from build123d import *

# Parameters (mm, degrees)
F1_DEPTH = 9.525
F3_D     = 2.7178


with BuildPart() as f1:
    # F0 (on Top) → F1 (new body)
    with BuildSketch(Plane.XY):
        with BuildLine():
            Line((161.925, -95.25), (161.925, 95.25))
            ThreePointArc((161.925, 95.25), (160.065128, 99.740128), (155.575, 101.6))
            Line((155.575, 101.6), (34.925, 101.6))
            ThreePointArc((34.925, 101.6), (30.434872, 99.740128), (28.575, 95.25))
            Line((28.575, 95.25), (28.575, 63.5))
            ThreePointArc((28.575, 63.5), (13.696024, 27.578976), (-22.225, 12.7))
            Line((-22.225, 12.7), (-155.575, 12.7))
            ThreePointArc((-155.575, 12.7), (-160.065128, 10.840128), (-161.925, 6.35))
            Line((-161.925, 6.35), (-161.925, -95.25))
            ThreePointArc((-161.925, -95.25), (-160.065128, -99.740128), (-155.575, -101.6))
            Line((-155.575, -101.6), (155.575, -101.6))
            ThreePointArc((155.575, -101.6), (160.065128, -99.740128), (161.925, -95.25))
        make_face()
        with BuildLine():
            Line((47.371, 9.652), (142.875, 9.652))
            ThreePointArc((142.875, 9.652), (145.030261, 8.759261), (145.923, 6.604))
            Line((145.923, 6.604), (145.923, -22.352))
            ThreePointArc((145.923, -22.352), (145.030261, -24.507261), (142.875, -25.4))
            Line((142.875, -25.4), (47.371, -25.4))
            ThreePointArc((47.371, -25.4), (45.215739, -24.507261), (44.323, -22.352))
            Line((44.323, -22.352), (44.323, 6.604))
            ThreePointArc((44.323, 6.604), (45.215739, 8.759261), (47.371, 9.652))
        make_face(mode=Mode.SUBTRACT)
    extrude(amount=-F1_DEPTH)

    # F3 (through all)
    with Locations(Plane.XY):
        with Locations((118.999, -56.134), (118.999, 14.732), (118.999, 68.834), (71.247, 68.834), (71.247, 14.732), (71.247, -56.134), (21.717, -60.706), (21.717, -91.44), (-3.683, -60.706), (-3.683, -91.44), (-29.083, -60.706), (-29.083, -91.44), (-54.483, -91.44), (-54.483, -60.706), (-66.929, -52.832), (-66.929, -21.082), (-92.329, -52.832), (-92.329, -21.082), (-124.079, -52.832), (-124.079, -21.082), (-149.479, -52.832), (-149.479, -21.082)):
            Hole(F3_D / 2)


solid = f1.part
Input: part model. Units: mm. Frame: model coordinates. A direction names the side the tool comes from. Give positions to 0.01 mm unless a question says otherwise; leave off trailing zeros. Loops run counter-clockwise (first coordinate to the right, second up) from the corner with the lowest first, then second, coordinate; pieces in that order, holes last. Notation, with made-up numbers: (61, 6.25) -> (109, 6.25) arc R11 cw to (109, 13.25) -> close; hole circle Ø11 at (-23, 74.5). An arc over 180 degrees is marked (long way). Answer as a JSON object with one key per item and string values. Group by question number.
Item 1: Line query: probe 1 along X at (y, z) = (-56, -7.25) (3 decimals); probe 2 along Y at (x, z) = (132, -4.75); probe 3 along X at (y, z) = (-10, -5.75) (3 decimals). Output: solid intervals per line, ascending.
Item 2: Pull-direction query (X, two-part tool) for faces 1 (the cylindrical face through (30.485, 99.789, -4.696)), 2 (the flat face through (-88, 12.7, -5)), 3 (the flat face through (145.923, -8, -5)), 4 (the cylindrical face through (160.114, 99.69, -4.696)); classes: released by +X, released by -X, zero draft, split by the parting line, or undercut.
Item 3: Cut plane C-C, the plane z = -8. State how many separate pieces and enclosed holes the cut face has, and give its area (3 significant figures).
Item 4: Cut plane B-B, the plane x = -116. Return the cut outline in (y, z) (3 decimals), and give its area (3 significant figures).
Item 5: Cut plane A-A, the plane x = 133.5. Return the cut outline in (y, z) (3 decimals), and give its area (3 significant figures).
Item 6: Cut plane D-D, the plane y = 24.5. Return the cut outline in (x, z) (3 decimals), and give its area (3 significant figures).
Item 7: Reachability of faces 5 (the flat face through (28.575, 80, -5)), 6 (the flat face through (44.323, -8, -5)), 7 (the flat face through (-2, -101.6, -5)) from +Z, -Z, +X, -X, +Y, -Y: full face, straight path, thin tool, end or side. Return the list, or none.
Item 8: Pin query (flat end, axial travel): P1, Ø3, axis at x = -119, z = -5.5, coming from the +Y side; P2, Ø1.5, axis at x = 31.5, z = -6.5, coming from the +Y side. Return the tip coordinate at first contact, or that it passes through.
Checks:
{
 "1": {"probe 1": "x = -161.925 to 69.895, 72.599 to 117.647, 120.351 to 161.925", "probe 2": "y = -101.6 to -25.4, 9.65 to 101.6", "probe 3": "x = -161.925 to 44.323, 145.923 to 161.925"},
 "2": {"face 1": "released by -X", "face 2": "zero draft", "face 3": "undercut", "face 4": "released by +X"},
 "3": {"separate pieces": "1", "enclosed holes": "23", "area": "45,700 mm²"},
 "4": {"outline": "(-101.6, -9.525) -> (12.7, -9.525) -> (12.7, 0) -> (-101.6, 0) -> close", "area": "1,090 mm²"},
 "5": {"outline": "(-101.6, -9.525) -> (-25.4, -9.525) -> (-25.4, 0) -> (-101.6, 0) -> close; (9.652, -9.525) -> (101.6, -9.525) -> (101.6, 0) -> (9.652, 0) -> close", "area": "1,600 mm²"},
 "6": {"outline": "(10.327, -9.525) -> (161.925, -9.525) -> (161.925, 0) -> (10.327, 0) -> close", "area": "1,440 mm²"},
 "7": {"face 5": "+Z, -Z, -X, +Y", "face 6": "+Z, -Z", "face 7": "+Z, -Z, +X, -X, -Y"},
 "8": {"P1": "stops at y = 12.7", "P2": "stops at y = 101.01"}
}
